from build123d import *

# Parameters (mm, degrees)
SKETCH1_R           = 7.5
BOSS_EXTRUDE1_DEPTH = 38
SKETCH2_R           = 20
BOSS_EXTRUDE2_DEPTH = 10
SKETCH3_R           = 15
BOSS_EXTRUDE3_DEPTH = 40


with BuildPart() as part:
    # Sketch1 → Boss-Extrude1 (new body)
    with BuildSketch(Plane(origin=(0, 0, 0), x_dir=(1, 0, 0), z_dir=(0, 1, 0))):
        with Locations(Location((0, 0, 0), (0, 0, 270))):
            Circle(SKETCH1_R)
    extrude(amount=BOSS_EXTRUDE1_DEPTH)

    # Sketch2 → Boss-Extrude2 (add)
    with BuildSketch(Plane.XZ):
        with Locations(Location((0, 0, 0), (0, 0, 270))):
            Circle(SKETCH2_R)
    extrude(amount=BOSS_EXTRUDE2_DEPTH)

    # Sketch3 → Boss-Extrude3 (add)
    with BuildSketch(Plane(origin=(0, 38, 0), x_dir=(1, 0, 0), z_dir=(0, 1, 0))):
        with Locations(Location((0.670369296, 0, 0), (0, 0, 270))):
            Circle(SKETCH3_R)
    extrude(amount=BOSS_EXTRUDE3_DEPTH)


solid = part.part
Check sheet for the modelled part. Datum: model origin and axes. Units: mm. A direction names the side the tool comes from. Round coordinates to 2 decimals unless told otherwise and drop trailing zeros. Write each loop counter-clockwise with the first axis right and the second up, starting at its lowest first coordinate (ties: lowest second). Pieces come first, ordered by that corner, then holes. Notation, with made-up numbers: (46, -15.75) -> (93, -15.75) arc R9 ccw to (93, -0.75) -> close; hole circle Ø9 at (-16, -1). An arc over 180 degrees is marked (long way). Answer as CSV lines item,"result". Start each with the question number.
1) Material ranges on line 1 (Y direction, x = -10, z = -4.5); line 2 (Y direction, x = -8, z = 15); line 3 (X direction, y = 61, z = -4.5), recorded low to high. Write a range as from..to.
2) Release check for a two-part mould opening along Y. For faces 1 (the flat face through (1, 78, 0)), 2 (the flat face through (0, -10, 0)), 3 (the cylindrical face through (0.33, 18.734, -7.493)) record: pulls with the +Y half, pulls with the -Y half, needs draft (parallel to the pull), parting line crosses it, or undercut.
3) Section check B-B on x = 9. Enter the section's corners in (y, z), and give its area (3 significant figures).
4) Section check A-A on z = -13.5. Enter the section's corners in (x, y), and give its area (3 significant figures).
5) Tool access check on faces 4 (the cylindrical face through (-13.973, 57.72, -3.252)), 5 (the cylindrical face through (-19.524, -4.93, 4.336)), 6 (the flat face through (0, 0, -9)). Record the directions out of +Z, -Z, +X, -X, +Y, -Y that give a thin tool (end or side, any length) a straight path to the whole face; none if there is none.
6) Section check D-D on y = 22. Enter the section's corners in (x, z).
7) Section check C-C on z = 0. Enter the section's corners in (x, y), and give its area (3 significant figures).
8) Go/stop test with flat-tipped pins: P1, Ø3, axis at y = 43.5, z = 7, coming from the -X side; P2, Ø2, axis at x = 8.5, y = 38.5, coming from the -Z side (3 decimals); P3, Ø4, axis at x = -0.5, y = 19, coming from the -Z side. Record where each tip stops, or that it passes through.
Found:
1,line 1,"y = -10..0, 38..78"
1,line 2,"y = -10..0"
1,line 3,"x = -13.64..14.98"
2,face 1,"pulls with the +Y half"
2,face 2,"pulls with the -Y half"
2,face 3,"undercut"
3,outline,"(-10, -17.86) -> (0, -17.86) -> (0, 17.86) -> (-10, 17.86) -> close; (38, -12.47) -> (78, -12.47) -> (78, 12.47) -> (38, 12.47) -> close"
3,area,"1,360 mm^2"
4,outline,"(-14.76, -10) -> (14.76, -10) -> (14.76, 0) -> (-14.76, 0) -> close; (-5.87, 38) -> (7.21, 38) -> (7.21, 78) -> (-5.87, 78) -> close"
4,area,"818 mm^2"
5,face 4,"+Y"
5,face 5,"+Y, -Y"
5,face 6,"none"
6,outline,"circle Ø15 at (0, 0)"
7,outline,"(-20, -10) -> (20, -10) -> (20, 0) -> (7.5, 0) -> (7.5, 38) -> (15.67, 38) -> (15.67, 78) -> (-14.33, 78) -> (-14.33, 38) -> (-7.5, 38) -> (-7.5, 0) -> (-20, 0) -> close"
7,area,"2,170 mm^2"
8,P1,"stops at x = -13.28"
8,P2,"stops at z = -13.355"
8,P3,"stops at z = -7.5"
